```python
from build123d import *

# Parameters (mm, degrees)
SKETCH_1_R          = 15
SKETCH_1_R_2        = 2
EXTRUDE_2_DEPTH     = 3
SKETCH_2_R          = 5
EXTRUDE_3_DEPTH     = 17
SKETCH_4_R          = 15
SKETCH_4_R_2        = 2
EXTRUDE_4_DEPTH     = 3
SKETCH_8_R          = 2
CUT_EXTRUDE_2_DEPTH = 15


with BuildPart() as part:
    # 草图1 → 凸台-拉伸2 (new body)
    with BuildSketch(Plane.XY):
        Circle(SKETCH_1_R)
        with Locations((10, 0)):
            Circle(SKETCH_1_R_2, mode=Mode.SUBTRACT)
        with Locations((-10, 0)):
            Circle(SKETCH_1_R_2, mode=Mode.SUBTRACT)
    extrude(amount=EXTRUDE_2_DEPTH)

    # 草图2 → 凸台-拉伸3 (add)
    with BuildSketch(Plane.XY.offset(3)):
        Circle(SKETCH_2_R)
    extrude(amount=EXTRUDE_3_DEPTH)

    # 草图4 → 凸台-拉伸4 (add)
    with BuildSketch(Plane.XY.offset(20)):
        Circle(SKETCH_4_R)
        with Locations((-10, 0)):
            Circle(SKETCH_4_R_2, mode=Mode.SUBTRACT)
        with Locations((0, 10)):
            Circle(SKETCH_4_R_2, mode=Mode.SUBTRACT)
        with Locations((10, 0)):
            Circle(SKETCH_4_R_2, mode=Mode.SUBTRACT)
        with Locations((0, -10)):
            Circle(SKETCH_4_R_2, mode=Mode.SUBTRACT)
    extrude(amount=EXTRUDE_4_DEPTH)

    # 草图8 → 切除-拉伸2 (cut)
    with BuildSketch(Plane.XY.offset(23)):
        Circle(SKETCH_8_R)
    extrude(amount=-CUT_EXTRUDE_2_DEPTH, mode=Mode.SUBTRACT)


solid = part.part
```
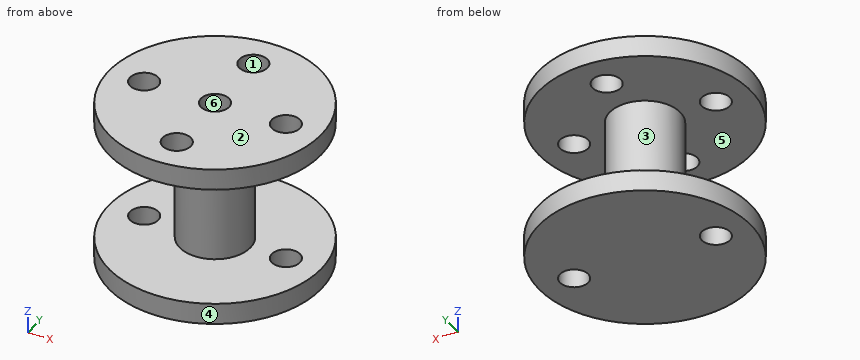
Input: part model. Units: mm. Frame: model coordinates. Face numbers are marked on the shaded views. A direction names the side the tool comes from. Give positions to 0.01 mm unless a question says otherwise; leave off trailing zeros. Order: outer loops, then holes, each group sorted by start corner. A loop starts at its lowest first (then second) coordinate and runs counter-clockwise, first axis right, second up. Notation, with made-up numbers: M 49,15 L 84,15 A24 ccw 84,43 Z; hole C 37.5,75.5 d4. An arc over 180 degrees is marked long. One line per question, with ' | ' between items. Start each with the question number.
1. Access query for the marked faces 1, 2 and 3. Directions: +Z, -Z, +X, -X, +Y, -Y. A direction counts if a zero-diameter tool reaches every point of the face in a straight line with its end or side. Return the directions, or none.
2. Pull-direction query (X, two-part tool) for the marked faces 4, 5 and 6; classes: released by +X, released by -X, zero draft, split by the parting line, or undercut.
3. Material intervals for probe 1 along Y at (x, z) = (0, 21.7); probe 2 along Z at (x, y) = (7.5, -11.25); probe 3 along Y at (x, z) = (0, 13.75), sorted ascending. Write a range as [from, to].
4. First-contact query: pin 1 Ø1 at (y, z) = (1, 14) entering from +X; pin 2 Ø6.5 at (x, y) = (-10, 0) entering from -Z; pin 3 Ø3 at (x, y) = (-10, 0) entering from -Z; pin 4 Ø1.5 at (y, z) = (-4.5, 6.5) entering from -X. Flat tips, straight axial feed; report the tip coordinate or a pass-through.
5. Section query B-B (x = 0). Return the cut outline in (y, z), and give its area (3 significant figures).
6. Section query C-C (y = 10). Return the cut outline in (x, z).
7. Section query A-A (y = 0). Count the separate pieces of the cut face and the enclosed holes in it, and give its area (3 significant figures).
8. Section query D-D (x = 10). Return the cut outline in (y, z), and give its area (3 significant figures).
Here are the results:
1) face 1: +Z | face 2: +Z, +X, -X, +Y, -Y | face 3: none
2) face 4: split by the parting line | face 5: zero draft | face 6: undercut
3) probe 1: [-15, -12], [-8, -2], [2, 8], [12, 15] | probe 2: [0, 3], [20, 23] | probe 3: [-5, -2], [2, 5]
4) pin 1: x = 4.97 | pin 2: z = 0 | pin 3: through | pin 4: x = -3.31
5) outline: M -15,0 L 15,0 L 15,3 L 5,3 L 5,20 L 8,20 L 8,23 L 2,23 L 2,8 L -2,8 L -2,23 L -8,23 L -8,20 L -5,20 L -5,3 L -15,3 Z; M -15,20 L -12,20 L -12,23 L -15,23 Z; M 12,20 L 15,20 L 15,23 L 12,23 Z | area: 266 mm²
6) outline: M -11.18,0 L 11.18,0 L 11.18,3 L -11.18,3 Z; M -11.18,20 L -2,20 L -2,23 L -11.18,23 Z; M 2,20 L 11.18,20 L 11.18,23 L 2,23 Z
7) separate pieces: 5 | enclosed holes: 0 | area: 242 mm²
8) outline: M -11.18,0 L -2,0 L -2,3 L -11.18,3 Z; M -11.18,20 L -2,20 L -2,23 L -11.18,23 Z; M 2,0 L 11.18,0 L 11.18,3 L 2,3 Z; M 2,20 L 11.18,20 L 11.18,23 L 2,23 Z | area: 110 mm²
